Source: three-view drawing plus pictorial views. Frame: mm from the lowest corner of the part. Give positions to 0.01 mm unless a question says otherwise; leave off trailing zeros. Write each loop counter-clockwise with the first axis right and the second up, starting at its lowest first coordinate (ties: lowest second). Pieces come first, ordered by that corner, then holes. Notation, with made-up numbers: M 43.5,-29.75 L 61.5,-29.75 A19 cw 61.5,-13.75 Z; hole C 26,34 d10. An arc over 180 degrees is marked long. Return JSON: item names as keys, results as strings.
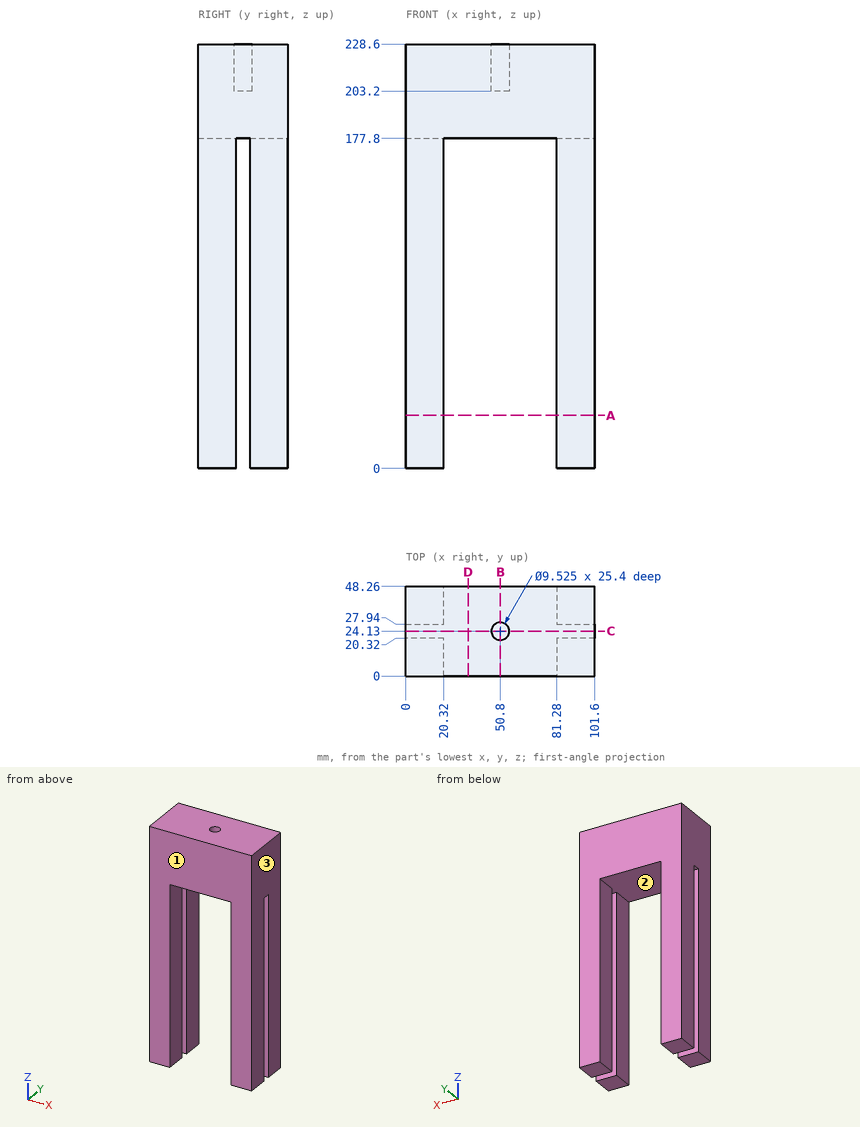
1) Cut plane C-C, the plane y = 24.13. Return the cut outline in (x, z), then the cut area to 3 significant figures.
Numbers:
{"outline": "M 0,177.8 L 101.6,177.8 L 101.6,228.6 L 55.56,228.6 L 55.56,203.2 L 46.04,203.2 L 46.04,228.6 L 0,228.6 Z", "area": "4,920 mm²"}
2) Contact query for a flat-ended pin moving along its axis: pin 1 Ø5 at (x, y) = (77.5, 14) entering from -Z. Output: stop coordinate, or through.
Numbers:
{"pin 1": "stops at z = 177.8"}
3) Draft query along X for the marked faces 1, 2 and 3. Return one class per face: released by +X, released by -X, zero draft, split by the parting line, or undercut.
Numbers:
{"face 1": "zero draft", "face 2": "undercut", "face 3": "released by +X"}
4) Cut plane D-D, the plane x = 33.5. Return the cut outline in (y, z).
Numbers:
{"outline": "M 0,177.8 L 48.26,177.8 L 48.26,228.6 L 0,228.6 Z"}
5) Cut plane B-B, the plane x = 50.8. Return the cut outline in (y, z).
Numbers:
{"outline": "M 0,177.8 L 48.26,177.8 L 48.26,228.6 L 28.89,228.6 L 28.89,203.2 L 19.37,203.2 L 19.37,228.6 L 0,228.6 Z"}
6) Line query: line 1 (Y direction, x = 89, z = 88); line 2 (X direction, y = 42.5, z = 116); line 3 (Y direction, x = 50.8, z = 213.25). Output: solid intervals per line, ascending. Write a range as [from, to].
Numbers:
{"line 1": "y = [0, 20.32], [27.94, 48.26]", "line 2": "x = [0, 20.32], [81.28, 101.6]", "line 3": "y = [0, 19.37], [28.89, 48.26]"}
7) Cut plane A-A, the plane z = 28.5. Return the cut outline in (x, y), then the cut area to 3 significant figures.
Numbers:
{"outline": "M 0,0 L 20.32,0 L 20.32,20.32 L 0,20.32 Z; M 0,27.94 L 20.32,27.94 L 20.32,48.26 L 0,48.26 Z; M 81.28,0 L 101.6,0 L 101.6,20.32 L 81.28,20.32 Z; M 81.28,27.94 L 101.6,27.94 L 101.6,48.26 L 81.28,48.26 Z", "area": "1,650 mm²"}
